Input: part model. Units: mm. Frame: model coordinates. A direction names the side the tool comes from. Give positions to 0.01 mm unless a question says otherwise; leave off trailing zeros. Loops run counter-clockwise (first coordinate to the right, second up) from the corner with the lowest first, then second, coordinate; pieces in that order, holes last. Notation, with made-up numbers: (-38, -9.5) - (15, -9.5) arc R19 cw to (15, 5.5) - close; hole circle Ø6 at (51.25, 63). An arc over 180 degrees is marked (long way). Answer as a JSON object with one key per item and string values.
from build123d import *

# Parameters (mm, degrees)
F1_DEPTH      = 64
F2_R          = 5
F3_R          = 10
F5_R          = 1.5
F6_DEPTH      = 32
F7_R          = 5
F9_DEPTH      = 10
F9_DEPTH_BACK = 15


with BuildPart() as f1:
    # F0 (on Front) → F1 (new body)
    with BuildSketch(Plane.XZ):
        with BuildLine():
            Line((0, 12.5), (0, 0))
            Line((0, 0), (17.5, 0))
            ThreePointArc((17.5, 0), (35, 17.5), (52.5, 0))
            Line((52.5, 0), (107.5, 0))
            ThreePointArc((107.5, 0), (125, 17.5), (142.5, 0))
            Line((142.5, 0), (160, 0))
            Line((160, 0), (160, 25))
            Line((160, 25), (35, 25))
            ThreePointArc((35, 25), (16.4174140659, 21.7812406156), (0, 12.5))
        make_face()
    extrude(amount=-F1_DEPTH)

    # F2
    f2_edges = [f1.edges().sort_by_distance(p)[0] for p in [
        (160, 32, 25),
        (0, 32, 0),
        (160, 32, 0),
    ]]
    fillet(f2_edges, radius=F2_R)

    # F3
    f3_edges = [f1.edges().sort_by_distance(p)[0] for p in [
        (0, 32, 12.5),
    ]]
    fillet(f3_edges, radius=F3_R)

    # F5 (on offset) → F6 (join)
    with BuildSketch(Plane.XZ.offset(-16)):
        with BuildLine():
            Line((17.5, 0), (52.5, 0))
            ThreePointArc((52.5, 0), (52.4351146235, 1.5055823014), (52.2409396496, 3))
            Line((52.2409396496, 3), (37.4494897428, 3))
            ThreePointArc((37.4494897428, 3), (35, 5), (32.5505102572, 3))
            Line((32.5505102572, 3), (17.7590603504, 3))
            ThreePointArc((17.7590603504, 3), (17.5648853765, 1.5055823014), (17.5, 0))
        make_face()
        with Locations((35, 2.5)):
            Circle(F5_R, mode=Mode.SUBTRACT)
        with BuildLine():
            Line((107.5, 0), (142.5, 0))
            ThreePointArc((142.5, 0), (125, 17.5), (107.5, 0))
        make_face()
        with Locations((125, 2.5)):
            Circle(F5_R, mode=Mode.SUBTRACT)
    extrude(amount=-F6_DEPTH)

    # F7
    f7_edges = [f1.edges().sort_by_distance(p)[0] for p in [
        (37.44949, 32, 3),
        (32.55051, 32, 3),
    ]]
    fillet(f7_edges, radius=F7_R)

    # F8 (on offset) → F9 (cut, two sides)
    with BuildSketch(Plane.XZ.offset(-16)) as f9_sk:
        with BuildLine():
            ThreePointArc((113.1874502253, 12.9117647059), (125, 4.5), (136.8125497747, 12.9117647059))
            ThreePointArc((136.8125497747, 12.9117647059), (125, 17.5), (113.1874502253, 12.9117647059))
        make_face()
        with BuildLine():
            ThreePointArc((113.1874502253, 12.9117647059), (125, 17.5), (136.8125497747, 12.9117647059))
            ThreePointArc((136.8125497747, 12.9117647059), (137.3269394455, 14.9271845456), (137.5, 17))
            ThreePointArc((137.5, 17), (122.9271845456, 29.3269394455), (113.1874502253, 12.9117647059))
        make_face()
    extrude(amount=-F9_DEPTH, mode=Mode.SUBTRACT)
    extrude(f9_sk.sketch, amount=F9_DEPTH_BACK, mode=Mode.SUBTRACT)


solid = f1.part
Item 1: Access query for faces 4 (the face through (159, 32, 23)), 5 (the face through (38.298, 32.224, 3.336)), 6 (the face through (124.615, 55.888, 17.496)), 7 (the face through (124.615, 0.777, 17.496)), 8 (the face through (1, 32, 2)). Directions: +Z, -Z, +X, -X, +Y, -Y. A direction counts if a zero-diameter tool reaches every point of the face in a straight line with its end or side. Return the directions, or none.
Geometry check:
{"face 4": "+Z, +X, +Y, -Y", "face 5": "+Y, -Y", "face 6": "-Z, +Y", "face 7": "-Z, -Y", "face 8": "-Z, -X, +Y, -Y"}
Item 2: Contact query for flat-ended pins moving along their axis: P1, Ø5.5, axis at x = 33.5, z = 2.5, coming from the +Y side; P2, Ø1.5, axis at x = 29.5, z = 3.5, coming from the -Y side; P3, Ø6, axis at x = 24.5, y = 37.5, coming from the +Z side. Output: stop coordinate, or through.
Geometry check:
{"P1": "stops at y = 48", "P2": "stops at y = 16", "P3": "stops at z = 24.49"}
Item 3: Mould query, pull axis Y, two halves, no side actions, for faces 1 (the face through (34.755, 16, 0.868)), 2 (the face through (125, 26, 15)), 3 (the face through (31.702, 32.224, 3.336)). Classes: released by +Y, released by -Y, zero draft, split by the parting line, or undercut.
Geometry check:
{"face 1": "released by -Y", "face 2": "undercut", "face 3": "zero draft"}
Item 4: Cut plane B-B (x = 28.5). Return loops of the section in (y, z).
Geometry check:
{"outline": "(0, 16.25) - (64, 16.25) - (64, 24.62) - (0, 24.62) - close; (16, 0) - (48, 0) - (48, 3) - (16, 3) - close"}
Item 5: Material intervals for line 1 (Z direction, x = 35, y = 34), sorted ascending. Write a range as [from, to].
Geometry check:
{"line 1": "z = [0, 1], [4, 5], [17.5, 25]"}
